from build123d import *

# Parameters (mm, degrees)
SKETCH_1_W      = 20
SKETCH_1_H      = 6
EXTRUDE_1_DEPTH = 1.5
FILLET_1_R      = 1.55


with BuildPart() as part:
    # 草图1 → 凸台-拉伸1 (new body)
    with BuildSketch(Plane(origin=(0, 0, 0), x_dir=(1, 0, 0), z_dir=(0, 1, 0))):
        with Locations((10, 3)):
            Rectangle(SKETCH_1_W, SKETCH_1_H)
        with BuildLine():
            Line((16.2, 1.45), (15.9, 1.45))
            ThreePointArc((15.9, 1.45), (14.35, 3), (15.9, 4.55))
            Line((15.9, 4.55), (16.2, 4.55))
            ThreePointArc((16.2, 4.55), (17.75, 3), (16.2, 1.45))
        make_face(mode=Mode.SUBTRACT)
        with BuildLine():
            Line((3.8, 1.45), (4.1, 1.45))
            ThreePointArc((4.1, 1.45), (5.65, 3), (4.1, 4.55))
            Line((4.1, 4.55), (3.8, 4.55))
            ThreePointArc((3.8, 4.55), (2.25, 3), (3.8, 1.45))
        make_face(mode=Mode.SUBTRACT)
    extrude(amount=EXTRUDE_1_DEPTH)

    # 圆角1
    fillet_1_edges = [part.edges().sort_by_distance(p)[0] for p in [
        (0, 0.75, -6),
        (20, 0.75, -6),
        (20, 0.75, 0),
        (0, 0.75, 0),
    ]]
    fillet(fillet_1_edges, radius=FILLET_1_R)


solid = part.part
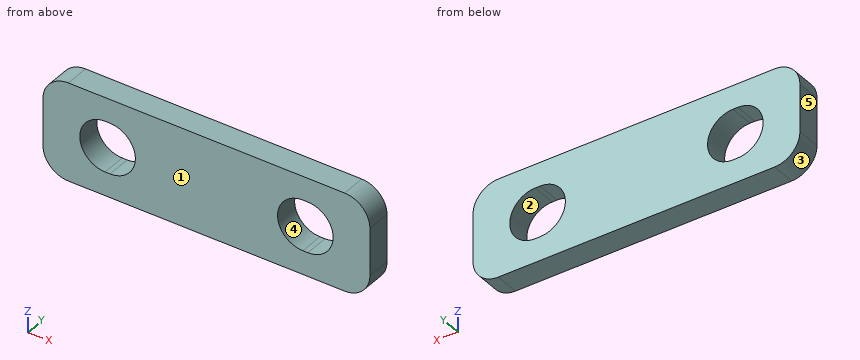
Verification items for the finished model (mm, model axes). Face numbers are marked on the shaded views. A direction names the side the tool comes from. Give positions to 0.01 mm unless a question says otherwise; leave off trailing zeros. Write each loop counter-clockwise with the first axis right and the second up, starting at its lowest first coordinate (ties: lowest second). Pieces come first, ordered by that corner, then holes.
(1) Cross-section at B-B (y = 0.4). Enter the section's corners in (x, z), plus the area to 3 significant figures.
(2) Mould release check, pull along Z, two halves, no side actions. Record for the marked faces 1, 2 and 3: +Z half, -Z half, draft (parallel to the pull), parting line (faces both ways), or undercut.
(3) Cross-section at C-C (x = 3). Enter the section's corners in (y, z), plus the area to 3 significant figures.
(4) Material ranges on line 1 (X direction, y = 0.3, z = -2.15); line 2 (X direction, y = 1.4, z = -2.7); line 3 (X direction, y = 1.05, z = -5), recorded low to high.
(5) Cross-section at D-D (z = -5.35). Enter the section's corners in (x, y), plus the area to 3 significant figures.
(6) Access from +Z, -Z, +X, -X, +Y, -Y to the whole of each face (thin tool, end or side, straight path). Record for the marked faces 4 and 5.
(7) Cross-section at A-A (z = -3). Enter the section's corners in (x, y).
(8) Gauge pin test, flat end, axial feed: pin 1 (1 mm diameter, centred on x = 3.5, z = -3.5, fed in from +Y). Record the tip position at first contact, or that the pin passes through.
Worked out:
1. outline: (0, -4.45) arc R1.55 ccw to (1.55, -6) - (18.45, -6) arc R1.55 ccw to (20, -4.45) - (20, -1.55) arc R1.55 ccw to (18.45, 0) - (1.55, 0) arc R1.55 ccw to (0, -1.55) - close; hole (3.8, -4.55) - (4.1, -4.55) arc R1.55 ccw to (4.1, -1.45) - (3.8, -1.45) arc R1.55 ccw to start; hole (15.9, -4.55) - (16.2, -4.55) arc R1.55 ccw to (16.2, -1.45) - (15.9, -1.45) arc R1.55 ccw to start
1. area: 101 mm2
2. face 1: draft
2. face 2: undercut
2. face 3: -Z half
3. outline: (0, -6) - (1.5, -6) - (1.5, -4.33) - (0, -4.33) - close; (0, -1.67) - (1.5, -1.67) - (1.5, 0) - (0, 0) - close
3. area: 5.02 mm2
4. line 1: x = 0 to 2.5, 5.4 to 14.6, 17.5 to 20
4. line 2: x = 0 to 2.28, 5.62 to 14.38, 17.72 to 20
4. line 3: x = 0.1 to 19.9
5. outline: (0.29, 0) - (19.71, 0) - (19.71, 1.5) - (0.29, 1.5) - close
5. area: 29.1 mm2
6. face 4: +Y, -Y
6. face 5: +Z, -Z, -X, +Y, -Y
7. outline: (0, 0) - (2.25, 0) - (2.25, 1.5) - (0, 1.5) - close; (5.65, 0) - (14.35, 0) - (14.35, 1.5) - (5.65, 1.5) - close; (17.75, 0) - (20, 0) - (20, 1.5) - (17.75, 1.5) - close
8. pin 1: passes through
